For this review, take the finished solid that the model builds, in its own axes (mm). A direction names the side the tool comes from. Round coordinates to 2 decimals unless told otherwise and drop trailing zeros. Write each loop counter-clockwise with the first axis right and the second up, starting at its lowest first coordinate (ties: lowest second). Pieces come first, ordered by that corner, then holes. Notation, with made-up numbers: M -35,-4.5 L -29,-4.5 A22 cw -29,18.5 Z; hole C 22.25,76 d3. An arc over 180 degrees is marked long. One line per question, with ' | ' between items.
```python
from build123d import *

# Parameters (mm, degrees)
SKETCH1_W                    = 90
SKETCH1_H                    = 25
BOSS_EXTRUDE1_DEPTH          = 16.87
SKETCH3_W                    = 10.75
SKETCH3_H                    = 10.75
CUT_EXTRUDE2_DEPTH           = 2.5
ENL_V_MAT_EXTRU_1_DEPTH      = 34
FILLET1_RADIUS               = 12.5
FILLET1_LENGTH               = 11.75
ESQUISSE5_R                  = 1.75
ENL_V_MAT_EXTRU_4_DEPTH      = 50.65729453
FILLET3_R                    = 4
SKETCH8_W                    = 38.029495875
SKETCH8_H                    = 20.943583685
CUT_EXTRUDE6_DEPTH           = 2
FILLET6_R                    = 2
FILLET7_R                    = 0.25
ESQUISSE17_R                 = 6.45
ENL_V_MAT_EXTRU_7_DEPTH      = 3.6
ENL_V_MAT_EXTRU_8_DEPTH      = 50.65729453
ENL_V_MAT_EXTRU_8_DEPTH_BACK = 50.65729453
ESQUISSE18_R                 = 50


with BuildPart() as part:
    # Sketch1 → Boss-Extrude1 (new body)
    with BuildSketch(Plane(origin=(0, 0, 0), x_dir=(1, 0, 0), z_dir=(0, 1, 0))):
        Rectangle(SKETCH1_W, SKETCH1_H)
    extrude(amount=BOSS_EXTRUDE1_DEPTH)

    # Sketch3 → Cut-Extrude2 (cut)
    with BuildSketch(Plane(origin=(0, 16.87, 0), x_dir=(1, 0, 0), z_dir=(0, 1, 0))):
        with Locations((-32.5, 0)):
            Rectangle(SKETCH3_W, SKETCH3_H)
    extrude(amount=-CUT_EXTRUDE2_DEPTH, mode=Mode.SUBTRACT)

    # Esquisse2 → Enlèv. mat.-Extru.1 (cut)
    with BuildSketch(Plane.XY.offset(12.5)):
        Polygon((45, 16.87), (10, 16.87), (19, 7.87), (45, 7.87), align=None)
        Polygon((-45, 0), (10, 0), (4.88, 5.12), (-45, 5.12), align=None)
    extrude(amount=-ENL_V_MAT_EXTRU_1_DEPTH, mode=Mode.SUBTRACT)

    # Fillet1: full round fillet: the end face becomes a half cylinder, R = half its width
    fillet1_face = Plane((-45, 10.995, 0), x_dir=(0, -1, 0), z_dir=(-1, 0, 0))  # on the end face: x along it, z out of the body
    fillet1_slab = fillet1_face.offset(-FILLET1_RADIUS / 2) * Box(FILLET1_LENGTH, 2 * FILLET1_RADIUS, FILLET1_RADIUS, mode=Mode.PRIVATE)  # the body's end, R deep
    fillet1_round = Plane((-32.5, 10.995, 0), x_dir=(-1, 0, 0), z_dir=(0, -1, 0)) * Cylinder(FILLET1_RADIUS, FILLET1_LENGTH, mode=Mode.PRIVATE)  # its axis R under the face
    add(fillet1_slab - fillet1_round, mode=Mode.SUBTRACT)

    # Esquisse5 → Enlèv. mat.-Extru.4 (cut, through all)
    with BuildSketch(Plane(origin=(0, 0, 0), x_dir=(-1, 0, 0), z_dir=(0, -1, 0))):
        with Locations(Location((-40, 0, 0), (0, 0, 90))):
            Circle(ESQUISSE5_R)
    extrude(amount=-ENL_V_MAT_EXTRU_4_DEPTH, mode=Mode.SUBTRACT)

    # Fillet3
    fillet3_edges = [part.edges().sort_by_distance(p)[0] for p in [
        (45, 3.935, -12.5),
        (45, 3.935, 12.5),
    ]]
    fillet(fillet3_edges, radius=FILLET3_R)

    # Sketch8 → Cut-Extrude6 (cut)
    with BuildSketch(Plane(origin=(0, 16.87, 0), x_dir=(1, 0, 0), z_dir=(0, 1, 0))):
        with Locations((-5.673362901, 3.675760168)):
            Rectangle(SKETCH8_W, SKETCH8_H)
    extrude(amount=-CUT_EXTRUDE6_DEPTH, mode=Mode.SUBTRACT)

    # Fillet6
    fillet6_edges = [part.edges().sort_by_distance(p)[0] for p in [
        (-24.688110839, 16.87, -2.851984162),
    ]]
    fillet(fillet6_edges, radius=FILLET6_R - 0.0001)  # a hair under: the kernel refuses the full size

    # Fillet7
    fillet7_edges = [part.edges().sort_by_distance(p)[0] for p in [
        (-37.875, 16.87, 0),
        (-32.5, 16.87, 5.375),
        (-27.125, 16.87, 0),
        (-32.5, 16.87, -5.375),
    ]]
    fillet(fillet7_edges, radius=FILLET7_R)

    # Esquisse17 → Enlèv. mat.-Extru.7 (cut)
    with BuildSketch(Plane.XZ.offset(-5.12)):
        with Locations((-32.5, 0)):
            Circle(ESQUISSE17_R)
    extrude(amount=-ENL_V_MAT_EXTRU_7_DEPTH, mode=Mode.SUBTRACT)

    # Esquisse18 → Enlèv. mat.-Extru.8 (cut, two sides: drawn at the far end of the back side and taken through both)
    with BuildSketch(Plane(origin=(0, 0, 0), x_dir=(1, 0, 0), z_dir=(0, 1, 0)).offset(-ENL_V_MAT_EXTRU_8_DEPTH_BACK)):
        with Locations((0, -50)):
            Circle(ESQUISSE18_R)
    extrude(amount=ENL_V_MAT_EXTRU_8_DEPTH + ENL_V_MAT_EXTRU_8_DEPTH_BACK, mode=Mode.SUBTRACT)


solid = part.part
```
Item 1: Machinability: for faces 1 (the face through (-33, 16, -5.375)), 2 (the face through (-26.35, 6.89, 1.94)), 3 (the face through (-7, 14.87, -5)), which of the approach directions +Z, -Z, +X, -X, +Y, -Y give a long, thin tool a straight path to every point of the face, cutting with its end or side? Answer none if there is none.
Results:
face 1: +Y | face 2: -Y | face 3: +Z, -Z, +X, +Y
Item 2: To check wall thickness, follow line 1 along Z through (x, y) = (-32.5, 7.1); line 2 along Z through (x, y) = (1, 6.75); line 3 along Y through (x, z) = (21.5, 4.25). State the ranges of each line that lie inside material, in increasing order. Write a range as from..to.
Results:
line 1: -12.5..-6.45, 6.45..12 | line 2: -12.5..0.01 | line 3: 0..7.87
Item 3: Mouldability with a two-part tool opening along X and no side actions: class faces 4 (the face through (43.797, 3.99, -11.359)), 5 (the face through (-20, 5.12, -3)), 6 (the face through (-27.125, 16, 0)) as +X half, -X half, draft (parallel to the pull), parting line (faces both ways), or undercut.
Results:
face 4: +X half | face 5: draft | face 6: undercut
Item 4: Take a section at A-A (x = 40). Write out the cut boundary in (y, z), then the cut area to 3 significant figures.
Results:
outline: M 0,-12.5 L 7.87,-12.5 L 7.87,-1.75 L 0,-1.75 Z; M 0,1.75 L 7.87,1.75 L 7.87,12.5 L 0,12.5 Z | area: 169 mm2
Item 5: Take a section at B-B (y = 1.75). Write out the cut boundary in (x, z), then the cut area to 3 significant figures.
Results:
outline: M 8.25,-12.5 L 41,-12.5 A4 ccw 45,-8.5 L 45,8.5 A4 ccw 41,12.5 L 33.07,12.5 A50 cw 8.25,0.69 Z; hole C 40,0 d3.5 | area: 720 mm2
Item 6: Insertion check: pin 1 Ø1.8 at (y, z) = (15.5, -2) entering from +X; pin 2 Ø1.8 at (x, y) = (-30, 15) entering from +Z; pin 3 Ø12.5 at (x, z) = (-29, 1) entering from -Y. Each pin has a flat end and moves straight along its axis. Give the tip position at first contact, or say it passes through.
Results:
pin 1: x = 12.27 | pin 2: z = 10.69 | pin 3: y = 5.12
Item 7: Take a section at D-D (x = 30). Write out the cut boundary in (y, z).
Results:
outline: M 0,-12.5 L 7.87,-12.5 L 7.87,10 L 0,10 Z
